Geometry: final body of the model. Coordinates: model frame, mm. A direction names the side the tool comes from. Round coordinates to 2 decimals unless told otherwise and drop trailing zeros. Loops run counter-clockwise (first coordinate to the right, second up) from the corner with the lowest first, then second, coordinate; pieces in that order, holes last. Notation, with made-up numbers: (2, 68.5) -> (29, 68.5) arc R38 ccw to (29, 106.5) -> close; hole circle Ø11 at (81, 22.5). An arc over 180 degrees is marked (long way). Answer in a Markdown table with one row per item.
```python
from build123d import *

# Parameters (mm, degrees)
CIRPATTERN1_COUNT = 2
CIRPATTERN1_ANGLE = 90


# Read off the part's stored shape, not the designer's step: ThreadSchematic
with BuildPart() as part:
    # ThreadSchematic outline → ThreadSchematic (revolve)
    with BuildSketch(Plane.YX):
        with BuildLine():
            Line((0, 8.9662), (0, 0))
            ThreePointArc((0, 0), (2.106401342, 0.733321609), (3.302000001, 2.616200001))
            Line((3.302000001, 2.616200001), (1.7526, 2.6162))
            Line((1.7526, 2.6162), (1.7526, 8.9662))
            Line((1.7526, 8.9662), (0, 8.9662))
        make_face()
    revolve(axis=Axis((0, 0, 0), (1, 0, 0)))

    # Sketch3 → Cross section 0
    with BuildSketch(Plane(origin=(0, 0, 0), x_dir=(0, 0, -1), z_dir=(1, 0, 0))):
        with BuildLine():
            Line((0.4318, -2.1463), (-0.4318, -2.1463))
            Line((-0.4318, -2.1463), (-0.4318, 2.1463))
            Line((-0.4318, 2.1463), (0.4318, 2.1463))
            Line((0.4318, 2.1463), (0.4318, -2.1463))
        make_face()
    # Sketch4 → Cross section 1
    with BuildSketch(Plane(origin=(2.4384, 0, 0), x_dir=(0, 0, -1), z_dir=(1, 0, 0))):
        with BuildLine():
            Line((0.2159, -0.2159), (-0.2159, -0.2159))
            Line((-0.2159, -0.2159), (-0.2159, 0.2159))
            Line((-0.2159, 0.2159), (0.2159, 0.2159))
            Line((0.2159, 0.2159), (0.2159, -0.2159))
        make_face()
    cross = loft(mode=Mode.SUBTRACT)

    # CirPattern1: Cross ×2 about axis
    cirpattern1_axis = Axis((0, 0, 0), (1, 0, 0))
    for i in range(1, CIRPATTERN1_COUNT):
        add(cross.rotate(cirpattern1_axis, i * CIRPATTERN1_ANGLE / (CIRPATTERN1_COUNT - 1)), mode=Mode.SUBTRACT)


solid = part.part
```
Item 1: Section query C-C, the plane y = 3. Output: boundary loops of the cut face in (x, z), and give its area (3 significant figures).
Ans:
| item | result |
|---|---|
| outline | (2.62, -1.38) -> (2.62, 1.38) arc R1.58 ccw to start |
| area | 1.58 mm2 |
Item 2: Section query A-A, the plane x = 3.25. Output: boundary loops of the cut face in (y, z).
Ans:
| item | result |
|---|---|
| outline | circle Ø3.51 at (0, 0) |
Item 3: Set-up query: faces 1 (the flat face through (8.966, 0, 0)), 2 (the cylindrical face through (5.84, 1.67, 0.53)). Return all of +Z, -Z, +X, -X, +Y, -Y with unobstructed straight access to the full face (end or side cutting, diameter ignored); none if empty.
Ans:
| item | result |
|---|---|
| face 1 | +Z, -Z, +X, +Y, -Y |
| face 2 | +X |
Item 4: Section query B-B, the plane z = -2.25. Output: boundary loops of the cut face in (x, y), and give its area (3 significant figures).
Ans:
| item | result |
|---|---|
| outline | (2.62, -2.42) -> (2.62, 2.42) arc R2.54 ccw to start |
| area | 6.24 mm2 |
Item 5: Ray query, L1, parallel to Z at x = 7.75, y = 0; L2, parallel to Y at x = 1.25, z = 0.75; L3, parallel to X at y = 0.5, z = 3. Return the intervals inside material, ascending.
Ans:
| item | result |
|---|---|
| L1 | -1.75 to 1.75 |
| L2 | -2.52 to -0.32, 0.32 to 2.52 |
| L3 | 1.89 to 2.62 |
Item 6: First-contact query: P1, Ø1, axis at y = -1, z = 2, coming from the -X side; P2, Ø1, axis at x = 7.5, y = 0, coming from the -Z side. Flat tips, straight axial feed; report the tip coordinate or a pass-through.
Ans:
| item | result |
|---|---|
| P1 | x = 0.48 |
| P2 | z = -1.75 |
